Here's how the part is built. I have some questions about the finished solid (model axes, mm). Give positions to 0.01 mm unless a question says otherwise; leave off trailing zeros. Write each loop counter-clockwise with the first axis right and the second up, starting at its lowest first coordinate (ties: lowest second). Pieces come first, ordered by that corner, then holes. Notation, with made-up numbers: (14, 64.5) - (63, 64.5) arc R14 cw to (63, 79.5) - close; hole circle Ø5 at (66.5, -2). An arc over 180 degrees is marked (long way). One line per item, written item: value. Start each with the question number.
1) Imagine slicing it at A-A on x = 11. Write out the boundary of the cut face in (y, z).
2) Please list where these lines run through material, in increasing order: L1, parallel to Z at x = -18.2, y = 0.7; L2, parallel to Z at x = 20.5, y = 0.1; L3, parallel to Z at x = 18.2, y = 0.5. Write a range as [from, to].
3) I'm going to push flat-ended pins straight in: P1, Ø0.5, axis at y = 0.5, z = -24.5, coming from the -X side; P2, Ø0.5, axis at x = -0.5, y = 0.5, coming from the -Z side. Where does each tip first touch, or does it pass through?
4) Imagine slicing it at B-B on y = 0.6. Count the separate pieces of the cut face and the enclosed holes in it, plus the area to 3 significant figures.
5) Imagine slicing it at C-C on z = 14. Write out the boundary of the cut face in (x, y).
Autodesk Inventor part; units mm, degrees
ref_plane "YZ Plane" through (0, 0, 0) normal (1, 0, 0) x (0, 1, 0)
ref_plane "XZ Plane" through (0, 0, 0) normal (0, 1, 0) x (-1, 0, 0)
ref_plane "XY Plane" through (0, 0, 0) normal (0, 0, 1) x (1, 0, 0)
sketch "Sketch1" plane through (0, 0, 0) normal (0, 1, 0) x (-1, 0, 0)
  line L0 (-25, -25) -> (25, -25)
  line L1 (25, -25) -> (25, 25)
  line L2 (25, 25) -> (-25, 25)
  line L3 (-25, 25) -> (-25, -25)
  line L4 (-25, -25) -> (25, 25) construction
  line L5 (25, -25) -> (-25, 25) construction
  point P0 (0, 0)
  dimension "d0" = 50
  dimension "d1" = 50
extrude "Extrusion1" add sketch "Sketch1" along normal blind 1
sketch "Sketch2" plane through (0, 1, 0) normal (0, 1, 0) x (1, 0, 0)
  line L0 (25, -25) -> (25, -15)
  line L1 (25, -25) -> (25, 25)
  line L2 (25, -15) -> (23.4, -15)
  line L3 (23.4, -15) -> (23.4, -5)
  line L4 (23.4, -5) -> (25, -5)
  line L5 (25, -5) -> (25, 5)
  line L6 (25, 5) -> (23.4, 5)
  line L7 (23.4, 5) -> (23.4, 15)
  line L8 (23.4, 15) -> (25, 15)
  line L9 (25, 15) -> (25, 25)
  line L10 (27, 25) -> (27, -25)
  line L11 (27, -25) -> (25, -25)
  point P0 (0, 0)
  dimension "d4" = 1.6
  dimension "d5" = 10
  dimension "d6" = 10
extrude "Extrusion2" cut sketch "Sketch2" against normal blind 1
sketch "Sketch3" plane through (0, 1, 0) normal (0, 1, 0) x (1, 0, 0)
  line L0 (25, 25) -> (25, 24)
  line L1 (25, 24) -> (15, 24)
  line L2 (15, 24) -> (15, 25)
  line L3 (25, 25) -> (-25, 25)
  line L4 (15, 25) -> (5, 25)
  line L5 (5, 25) -> (5, 24)
  line L6 (5, 24) -> (-5, 24)
  line L7 (-5, 24) -> (-5, 25)
  line L8 (-5, 25) -> (-15, 25)
  line L9 (-15, 25) -> (-15, 24)
  line L10 (-15, 24) -> (-25, 24)
  line L11 (-25, 24) -> (-25, 27)
  line L12 (-25, 27) -> (25, 27)
  line L13 (25, 27) -> (25, 25)
  point P0 (0, 0)
extrude "Extrusion3" cut sketch "Sketch3" against normal blind 1
sketch "Sketch4" plane through (0, 1, 0) normal (0, 1, 0) x (1, 0, 0)
  line L0 (-25, -25) -> (-25, -15)
  line L1 (-25, -15) -> (-24, -15)
  line L2 (-24, -15) -> (-24, -5)
  line L3 (-24, -5) -> (-25, -5)
  line L4 (-25, 24) -> (-25, -25)
  line L5 (-25, -5) -> (-25, 5)
  line L6 (-25, 24) -> (-25, -25)
  line L7 (-25, 5) -> (-24, 5)
  line L8 (-24, 5) -> (-24, 15)
  line L9 (-24, 15) -> (-25, 15)
  line L10 (-25, 24) -> (-27, 23)
  line L11 (-27, 23) -> (-27, -24.2648)
  line L12 (-27, -24.2648) -> (-25, -25)
  point P0 (0, 0)
  dimension "d11" = 10
  dimension "d12" = 10
  dimension "d13" = 10
extrude "Extrusion4" cut sketch "Sketch4" against normal blind 1 contours L4 L3 L2 L1 | L4 L9 L8 L7
sketch "Sketch5" plane through (0, 1, 0) normal (0, 1, 0) x (1, 0, 0)
  line L0 (-25, -25) -> (-15, -25)
  line L1 (-25, -25) -> (25, -25)
  line L2 (-15, -25) -> (-15, -24)
  line L3 (-15, -24) -> (-5, -24)
  line L4 (-5, -24) -> (-5, -25)
  line L5 (-5, -25) -> (5, -25)
  line L6 (5, -25) -> (5, -24)
  line L7 (5, -24) -> (15, -24)
  line L8 (15, -24) -> (15, -25)
  line L9 (25, -25) -> (25, -26)
  line L10 (25, -26) -> (-25, -26)
  line L11 (-25, -26) -> (-25, -25)
  point P0 (0, 0)
  dimension "d16" = 10
extrude "Extrusion5" cut sketch "Sketch5" against normal blind 1 contours L2 L3 L4 L1 | L6 L7 L8 L1
sketch "Sketch6" plane through (0, 1, 0) normal (0, 1, 0) x (1, 0, 0)
  circle A0 centre (-21.5, -18.2) radius 0.5
  circle A1 centre (-18.2, 21.5) radius 0.5
  circle A2 centre (18.2, -21.5) radius 0.5
  circle A3 centre (21.5, 18.2) radius 0.5
  line L0 (15, -25) -> (25, -25)
  line L1 (25, -25) -> (25, -15)
  line L2 (-25, -25) -> (-15, -25)
  line L3 (-25, -15) -> (-25, -25)
  line L4 (-5, 25) -> (-15, 25)
  line L5 (-25, 24) -> (-25, 15)
  line L6 (25, 24) -> (15, 24)
  line L7 (25, 15) -> (25, 24)
  point P0 (0, 0)
  dimension "d21" = 1
  dimension "d22" = 1
  dimension "d23" = 1
  dimension "d24" = 1
  dimension "d25" = 3.5
  dimension "d26" = 6.8
  dimension "d27" = 6.8
  dimension "d28" = 3.5
  dimension "d29" = 3.5
  dimension "d30" = 6.8
  dimension "d31" = 5.8
  dimension "d32" = 3.5
extrude "Extrusion6" cut sketch "Sketch6" against normal blind 1
properties part number "Side Panel"
Numbers:
1. outline: (0, -25) - (1, -25) - (1, 24) - (0, 24) - close
2. L1: [-24, -22], [-21, 25]
2. L2: [-24, 25]
2. L3: [-24, 21], [22, 25]
3. P1: x = -15
3. P2: z = -24
4. separate pieces: 1
4. enclosed holes: 4
4. area: 2,390 mm^2
5. outline: (-24, 0) - (23.4, 0) - (23.4, 1) - (-24, 1) - close
